Autodesk Fusion 360 part; units mm, degrees
sketch "Sketch1" plane through (0, 0, 0) normal (0, 0, 1) x (1, 0, 0)
  circle A0 centre (0, 0) radius 35.5
  circle A1 centre (0, 0) radius 32.5
  dimension "d2" = 71
  dimension "d3" = 65
extrude "Extrude1" add sketch "Sketch1" along normal blind 14
sketch "Sketch2" plane through (0, 0, 0) normal (0, 0, 1) x (1, 0, 0)
  circle A0 centre (0, 0) radius 31
  dimension "d8" = 62
sketch "Sketch3" plane through (0, 0, 0) normal (0, 0, 1) x (1, 0, 0)
  circle A0 centre (0, 0) radius 32.5
  circle A1 centre (0, 0) radius 31.0483
extrude "Extrude3" add sketch "Sketch3" sketch "Sketch1" against normal blind 2.15 of sketch 2
fillet "Fillet1" radius 1 1 edges at (-33.0976, 12.8373, -2.15)
sketch "Sketch4" plane through (0, 0, 0) normal (0, 1, 0) x (1, 0, 0)
  line L0 (-35.5, -14) -> (35.5, -14)
  line L1 (0, -14) -> (0, -11)
  circle A0 centre (0, -10) radius 1
  dimension "d13" = 3
  dimension "d14" = 2
extrude "Extrude4" cut sketch "Sketch4" along normal through all and the other way through all
sketch "Sketch5" plane through (0, 0, 0) normal (1, 0, 0) x (0, 1, 0)
  line L0 (0, 14) -> (0, 11)
  circle A0 centre (0, 10) radius 1
  point P0 (0, 14)
  dimension "d16" = 3
  dimension "d17" = 2
extrude "Extrude5" cut sketch "Sketch5" along normal through all and the other way through all
ref_plane "WorkPlane1" through (0, 35.5, 0) normal (0, 1, 0) x (0, 0, 1)
sketch "Sketch6" plane through (0, 35.5, 0) normal (0, 1, 0) x (1, 0, 0)
  circle A0 centre (0, -10) radius 1.9
  dimension "d24" = 3.8
extrude "Extrude6" cut sketch "Sketch6" against normal blind 1.5
ref_plane "WorkPlane2" through (0, -35.5, 0) normal (0, 1, 0) x (0, 0, 1)
sketch "Sketch7" plane through (0, -35.5, 0) normal (0, 1, 0) x (1, 0, 0)
  circle A0 centre (0, -10) radius 1.9
  circle A1 centre (0, -10) radius 1
  dimension "d28" = 3.8
extrude "Extrude7" cut sketch "Sketch7" along normal blind 1.5
ref_plane "WorkPlane3" through (-35.5, 0, 0) normal (1, 0, 0) x (0, 1, 0)
sketch "Sketch8" plane through (-35.5, 0, 0) normal (1, 0, 0) x (0, 1, 0)
  circle A0 centre (0, 9.9) radius 1.9
  dimension "d32" = 3.8
extrude "Extrude8" cut sketch "Sketch8" along normal blind 1.5
ref_plane "WorkPlane4" through (35.5, 0, 0) normal (1, 0, 0) x (0, 1, 0)
sketch "Sketch9" plane through (35.5, 0, 0) normal (1, 0, 0) x (0, 1, 0)
  circle A0 centre (0, 9.9) radius 1.9
  circle A1 centre (0, 9.9) radius 1.9
  dimension "d36" = 3.8
extrude "Extrude9" cut sketch "Sketch9" against normal blind 1.5
fillet "Fillet3" radius 1 1 edges at (-33.0976, -12.8373, 14)
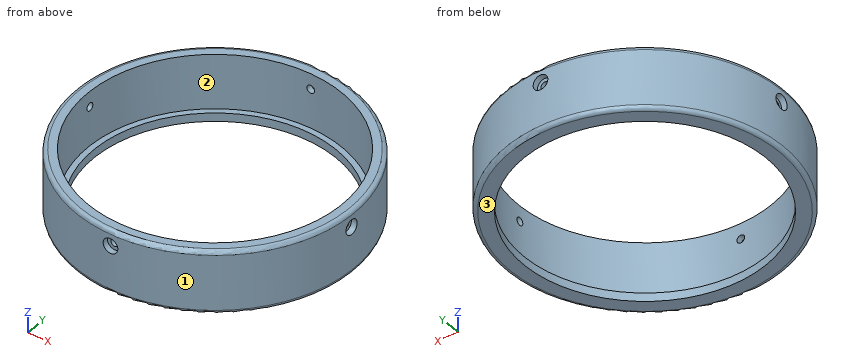
For this review, take the finished solid that the model builds, in its own axes (mm). Face numbers are marked on the shaded views. Coordinates: 2 decimals unless noted, no trailing zeros. Order: outer loops, then holes, each group sorted by start corner. A loop starts at its lowest first (then second) coordinate and runs counter-clockwise, first axis right, second up. Notation, with made-up numbers: (27.25, 30.5) - (73.25, 30.5) arc R16 cw to (73.25, 54.5) - close; hole circle Ø2 at (73, -17.5). An arc over 180 degrees is marked (long way). Use one line per item in the form item = value.
Q1. Consider section A-A (y = 0). Give the number of separate pieces and of enclosed holes in the cut face, then the cut area to 3 significant figures.
Checked values:
separate_pieces = 4
enclosed_holes = 0
area = 84.9 mm2
Q2. Draft analysis for pull direction X (two halves, no side actions). For the marked faces 1, 2 and 3, state which applies: +X half, -X half, draft (parallel to the pull), parting line (faces both ways), or undercut.
Checked values:
face_1 = parting line
face_2 = undercut
face_3 = draft
Q3. For P1, Ø4, axis at y = -18.5, z = 5, coming from the +X side; P2, Ø2, axis at x = 14.5, z = 2, coming from the -Y side; P3, Ø1.6, axis at y = 0, z = 10, coming from the -X side; P4, Ø5, axis at y = 9, z = 9.5, coming from the +X side, all flat-tipped, find the tip position at first contact; note any pin that passes through.
Checked values:
P1 = 31.43
P2 = -32.83
P3 = through
P4 = 34.9
Q4. For probe 1 along X at (y, z) = (13, 5); probe 2 along Y at (x, z) = (-20, 0.75); probe 3 along X at (y, z) = (0, 7.75), list the stretches that pass through material, from the lowest coordinate up. Write a range as from..to.
Checked values:
probe_1 = -33.03..-29.79, 29.79..33.03
probe_2 = -29.33..-25.62, 25.62..29.33
probe_3 = -35.5..-32.5, 32.5..35.5
Q5. Consider section C-C (z = 1.5). Give the boundary of the cut face in (x, y).
Checked values:
outline = circle Ø71 at (0, 0); hole circle Ø65 at (0, 0)
